For this review, use the dimensioned drawing (mm, ordinates from the lowest corner) and the shaded views. A direction names the side the tool comes from. Round coordinates to 2 decimals unless told otherwise and drop trailing zeros. Loops run counter-clockwise (first coordinate to the right, second up) from the corner with the lowest first, then second, coordinate; pieces in that order, holes last.
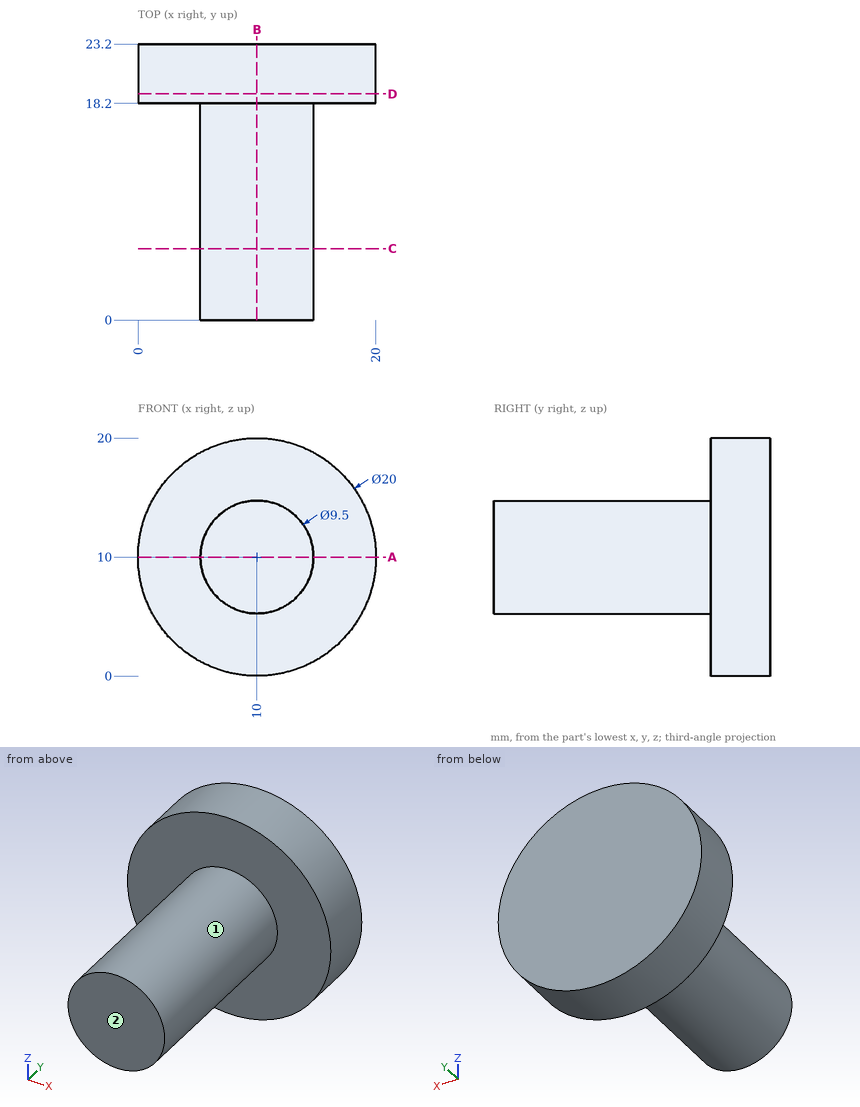
(1) Add section D-D (y = 19). Give the boundary of the cut face in (x, z).
(2) Add section C-C (y = 6). Give the boundary of the cut face in (x, z), plus the area to 3 significant figures.
(3) For the marked faces 1 and 2, list the 3-axis set-ups (+Z, -Z, +X, -X, +Y, -Y) from which the entire face can be reached by the end or side of a thin tool; tool diameter is ignored.
(4) Add section A-A (z = 10). Give the boundary of the cut face in (x, y), plus the area to 3 significant figures.
(5) For L1, parallel to Y at x = 4.25, z = 13; L2, parallel to Z at x = 10, y = 7.75, list the stretches that pass through material, from the lowest coordinate up.
(6) Add section B-B (x = 10). Give the boundary of the cut face in (y, z), plus the area to 3 significant figures.
(7) Insertion check: pin 1 Ø1.5 at (y, z) = (10, 11.5) entering from +X; pin 2 Ø5 at (x, y) = (16.5, 10.5) entering from -Z; pin 3 Ø1.5 at (y, z) = (5, 5) entering from -X. Each pin has a flat end and moves straight along its axis. Give the tip position at first contact, or say it passes through.
Outcome:
1. outline: circle Ø20 at (10, 10)
2. outline: circle Ø9.5 at (10, 10)
2. area: 70.9 mm2
3. face 1: -Y
3. face 2: +Z, -Z, +X, -X, -Y
4. outline: (0, 18.2) - (5.25, 18.2) - (5.25, 0) - (14.75, 0) - (14.75, 18.2) - (20, 18.2) - (20, 23.2) - (0, 23.2) - close
4. area: 273 mm2
5. L1: y = 18.2 to 23.2
5. L2: z = 5.25 to 14.75
6. outline: (0, 5.25) - (18.2, 5.25) - (18.2, 0) - (23.2, 0) - (23.2, 20) - (18.2, 20) - (18.2, 14.75) - (0, 14.75) - close
6. area: 273 mm2
7. pin 1: stops at x = 14.69
7. pin 2: stops at z = 7.44
7. pin 3: stops at x = 7.88
